Verification items for the finished model (mm, model axes). A direction names the side the tool comes from. Coordinates: 2 decimals unless noted, no trailing zeros. Order: outer loops, then holes, each group sorted by start corner. A loop starts at its lowest first (then second) coordinate and runs counter-clockwise, first axis right, second up. Notation, with made-up numbers: M 59,5 L 115,5 A26 cw 115,19 Z; hole C 47,13.25 d5. An arc over 180 degrees is marked long. Write item = value, one per line.
```python
from build123d import *

# Parameters (mm, degrees)
SKETCH_1_W           = 55
SKETCH_1_H           = 55
EXTRUDE_1_DEPTH      = 12
CUT_EXTRUDE_1_REACH  = 42.7
SKETCH_2_R           = 1.5
SKETCH_3_R           = 20
CUT_EXTRUDE_2_DEPTH  = 10
CUT_EXTRUDE_3_REACH  = 42.7
EXTRUDE_2_DEPTH      = 6
EXTRUDE_2_DEPTH_BACK = 15
SKETCH_5_R           = 2.25
SKETCH_6_W           = 14
SKETCH_6_H           = 14
EXTRUDE_3_DEPTH      = 1
SKETCH_7_R           = 3.5
EXTRUDE_4_DEPTH      = 0.5
SKETCH_8_W           = 30
SKETCH_8_H           = 30
EXTRUDE_5_DEPTH      = 0.1


with BuildPart() as part:
    # 草图1 → 凸台-拉伸1 (new body)
    with BuildSketch(Plane.XY):
        Rectangle(SKETCH_1_W, SKETCH_1_H)
    extrude(amount=EXTRUDE_1_DEPTH)

    # 草图2 → 切除-拉伸1 (cut, up to next)
    with BuildSketch(Plane.XY.offset(12), mode=Mode.PRIVATE) as cut_extrude_1_sk1:
        with Locations((21.5, 21.5)):
            Circle(SKETCH_2_R)
    cut_extrude_1_tool1 = extrude(cut_extrude_1_sk1.sketch, amount=-CUT_EXTRUDE_1_REACH, mode=Mode.PRIVATE) & part.part
    # 草图2 → 切除-拉伸1 (cut, up to next)
    with BuildSketch(Plane.XY.offset(12), mode=Mode.PRIVATE) as cut_extrude_1_sk2:
        with Locations((21.5, -21.5)):
            Circle(SKETCH_2_R)
    cut_extrude_1_tool2 = extrude(cut_extrude_1_sk2.sketch, amount=-CUT_EXTRUDE_1_REACH, mode=Mode.PRIVATE) & part.part
    # 草图2 → 切除-拉伸1 (cut, up to next)
    with BuildSketch(Plane.XY.offset(12), mode=Mode.PRIVATE) as cut_extrude_1_sk3:
        with Locations((-21.5, -21.5)):
            Circle(SKETCH_2_R)
    cut_extrude_1_tool3 = extrude(cut_extrude_1_sk3.sketch, amount=-CUT_EXTRUDE_1_REACH, mode=Mode.PRIVATE) & part.part
    # 草图2 → 切除-拉伸1 (cut, up to next)
    with BuildSketch(Plane.XY.offset(12), mode=Mode.PRIVATE) as cut_extrude_1_sk4:
        with Locations((-21.5, 21.5)):
            Circle(SKETCH_2_R)
    cut_extrude_1_tool4 = extrude(cut_extrude_1_sk4.sketch, amount=-CUT_EXTRUDE_1_REACH, mode=Mode.PRIVATE) & part.part
    add(cut_extrude_1_tool1.solids().sort_by_distance((21.5, 21.5, 12))[0], mode=Mode.SUBTRACT)
    add(cut_extrude_1_tool2.solids().sort_by_distance((21.5, -21.5, 12))[0], mode=Mode.SUBTRACT)
    add(cut_extrude_1_tool3.solids().sort_by_distance((-21.5, -21.5, 12))[0], mode=Mode.SUBTRACT)
    add(cut_extrude_1_tool4.solids().sort_by_distance((-21.5, 21.5, 12))[0], mode=Mode.SUBTRACT)

    # 草图3 → 切除-拉伸2 (cut)
    with BuildSketch(Plane.XY.offset(12)):
        Circle(SKETCH_3_R)
    extrude(amount=-CUT_EXTRUDE_2_DEPTH, mode=Mode.SUBTRACT)

    # 草图4 → 切除-拉伸3 (cut, up to next)
    with BuildSketch(Plane.XY.offset(12), mode=Mode.PRIVATE) as cut_extrude_3_sk1:
        Polygon((-27.5, 20.22970773), (-20.22970773, 27.5), (-27.5, 27.5), align=None)
    cut_extrude_3_tool1 = extrude(cut_extrude_3_sk1.sketch, amount=-CUT_EXTRUDE_3_REACH, mode=Mode.PRIVATE) & part.part
    # 草图4 → 切除-拉伸3 (cut, up to next)
    with BuildSketch(Plane.XY.offset(12), mode=Mode.PRIVATE) as cut_extrude_3_sk2:
        Polygon((20.22970773, -27.5), (27.5, -20.22970773), (27.5, -27.5), align=None)
    cut_extrude_3_tool2 = extrude(cut_extrude_3_sk2.sketch, amount=-CUT_EXTRUDE_3_REACH, mode=Mode.PRIVATE) & part.part
    # 草图4 → 切除-拉伸3 (cut, up to next)
    with BuildSketch(Plane.XY.offset(12), mode=Mode.PRIVATE) as cut_extrude_3_sk3:
        Polygon((20.22970773, 27.5), (27.5, 20.22970773), (27.5, 27.5), align=None)
    cut_extrude_3_tool3 = extrude(cut_extrude_3_sk3.sketch, amount=-CUT_EXTRUDE_3_REACH, mode=Mode.PRIVATE) & part.part
    # 草图4 → 切除-拉伸3 (cut, up to next)
    with BuildSketch(Plane.XY.offset(12), mode=Mode.PRIVATE) as cut_extrude_3_sk4:
        Polygon((-20.22970773, -27.5), (-27.5, -27.5), (-27.5, -20.22970773), align=None)
    cut_extrude_3_tool4 = extrude(cut_extrude_3_sk4.sketch, amount=-CUT_EXTRUDE_3_REACH, mode=Mode.PRIVATE) & part.part
    add(cut_extrude_3_tool1.solids().sort_by_distance((-25.076569, 25.076569, 12))[0], mode=Mode.SUBTRACT)
    add(cut_extrude_3_tool2.solids().sort_by_distance((25.076569, -25.076569, 12))[0], mode=Mode.SUBTRACT)
    add(cut_extrude_3_tool3.solids().sort_by_distance((25.076569, 25.076569, 12))[0], mode=Mode.SUBTRACT)
    add(cut_extrude_3_tool4.solids().sort_by_distance((-25.076569, -25.076569, 12))[0], mode=Mode.SUBTRACT)

    # 草图5 → 凸台-拉伸2 (add, two sides: drawn at the far end of the back side and taken through both)
    with BuildSketch(Plane.XY.offset(12).offset(-EXTRUDE_2_DEPTH_BACK)):
        with Locations((-25.5, 15.5)):
            Circle(SKETCH_5_R)
        with Locations((25.5, -15.5)):
            Circle(SKETCH_5_R)
    extrude(amount=EXTRUDE_2_DEPTH + EXTRUDE_2_DEPTH_BACK)

    # 草图6 → 凸台-拉伸3 (add)
    with BuildSketch(Plane(origin=(0, 0, 0), x_dir=(-1, 0, 0), z_dir=(0, 0, -1))):
        Rectangle(SKETCH_6_W, SKETCH_6_H)
    extrude(amount=EXTRUDE_3_DEPTH)

    # 草图7 → 凸台-拉伸4 (add)
    with BuildSketch(Plane(origin=(0, 0, -1), x_dir=(-1, 0, 0), z_dir=(0, 0, -1))):
        Circle(SKETCH_7_R)
    extrude(amount=EXTRUDE_4_DEPTH)

    # 草图8 → 凸台-拉伸5 (add)
    with BuildSketch(Plane(origin=(0, 0, 0), x_dir=(-1, 0, 0), z_dir=(0, 0, -1))):
        Rectangle(SKETCH_8_W, SKETCH_8_H)
    extrude(amount=EXTRUDE_5_DEPTH)


solid = part.part
```
Item 1: Sectioned sample at C-C, the plane y = 0. Enter the section's corners in (x, z), then the cut area to 3 significant figures.
Report:
outline = M -27.5,0 L -15,0 L -15,-0.1 L -7,-0.1 L -7,-1 L -3.5,-1 L -3.5,-1.5 L 3.5,-1.5 L 3.5,-1 L 7,-1 L 7,-0.1 L 15,-0.1 L 15,0 L 27.5,0 L 27.5,12 L 20,12 L 20,2 L -20,2 L -20,12 L -27.5,12 Z
area = 279 mm^2
Item 2: Gauge pin test, flat ends, axial feed: pin 1 (10 mm diameter, centred on x = -8, y = -13.5, fed in from +Z); pin 2 (1.8 mm diameter, centred on y = 18, z = 7, fed in from -X); pin 3 (6 mm diameter, centred on y = 8.5, z = 7, fed in from +X). Record the tip position at first contact, or that the pin passes through.
Report:
pin_1 = 12
pin_2 = -27.5
pin_3 = 27.5
Item 3: Scan lines: L1, parallel to Y at x = -21.5, z = 5.5; L2, parallel to Z at x = 16.5, y = 2.5; L3, parallel to X at y = -22.5, z = 1. Record each from-to range of solid material in increasing order. Write a range as from..to.
Report:
L1 = -26.23..-23, -20..20, 23..26.23
L2 = 0..2
L3 = -25.23..-22.62, -20.38..20.38, 22.62..25.23
Item 4: Release check for a two-part mould opening along X. For faces 1 (the flat face through (-26, 16, -3)), 2 (the flat face through (27.5, -18, 6)), 3 (the cylindrical face through (-22.61, -20.49, 6.08)), 4 (the flat face through (0, 0, 2)) record: pulls with the +X half, pulls with the -X half, needs draft (parallel to the pull), parting line crosses it, or undercut.
Report:
face_1 = needs draft
face_2 = pulls with the +X half
face_3 = undercut
face_4 = undercut
Item 5: Sectioned sample at A-A, the plane z = 9.25. Enter the section's corners in (x, y), then the cut area to 3 significant figures.
Report:
outline = M -27.5,-20.23 L -20.23,-27.5 L 20.23,-27.5 L 27.5,-20.23 L 27.5,-16.53 A2.25 ccw 27.5,-14.47 L 27.5,20.23 L 20.23,27.5 L -20.23,27.5 L -27.5,20.23 L -27.5,16.53 A2.25 ccw -27.5,14.47 Z; hole C -21.5,-21.5 d3; hole C -21.5,21.5 d3; hole C 0,0 d40; hole C 21.5,-21.5 d3; hole C 21.5,21.5 d3
area = 1,640 mm^2
Item 6: Sectioned sample at B-B, the plane x = 21.5. Enter the section's corners in (y, z).
Report:
outline = M -26.23,0 L -23,0 L -23,12 L -26.23,12 Z; M -20,0 L 20,0 L 20,12 L -20,12 Z; M 23,0 L 26.23,0 L 26.23,12 L 23,12 Z
Item 7: Tool access check on faces 5 (the flat face through (27.5, 3, 6)), 6 (the cylindrical face through (27.646, -14.824, 9.686)), 7 (the flat face through (3, 3, -1)). Record the directions out of +Z, -Z, +X, -X, +Y, -Y that give a thin tool (end or side, any length) a straight path to the whole face; none if there is none.
Report:
face_5 = +Z, -Z, +X, +Y
face_6 = none
face_7 = -Z
